```python
from build123d import *

# Parameters (mm, degrees)
SKETCH5_W           = 6.1595
SKETCH5_H           = 101.6
SKETCH5_W_2         = 101.6
SKETCH5_H_2         = 6.1595
BOSS_EXTRUDE1_DEPTH = 19.05
SKETCH6_W           = 333.025633445
SKETCH6_H           = 150.821732437
CUT_EXTRUDE1_DEPTH  = 205.486
SKETCH7_W           = 172.839732196
SKETCH7_H           = 155.996881263
CUT_EXTRUDE2_DEPTH  = 205.486
SKETCH8_W           = 181.528793167
SKETCH8_H           = 183.344081098
CUT_EXTRUDE3_DEPTH  = 147.066


with BuildPart() as part:
    # Sketch2 → Loft1 section 0
    with BuildSketch(Plane(origin=(0, 127, 0), x_dir=(1, 0, 0), z_dir=(0, 1, 0))):
        with BuildLine():
            Line((-50.8, -50.8), (278.13, -50.8))
            Line((278.13, -50.8), (278.13, 276.352))
            Line((278.13, 276.352), (-50.8, 276.352))
            Line((-50.8, 276.352), (-50.8, -50.8))
        make_face()
    # Sketch1 → Loft1 section 1
    with BuildSketch(Plane(origin=(0, 0, 0), x_dir=(1, 0, 0), z_dir=(0, 1, 0))):
        with BuildLine():
            Line((0, 0), (227.33, 0))
            Line((227.33, 0), (227.33, 225.552))
            Line((227.33, 225.552), (0, 225.552))
            Line((0, 225.552), (0, 0))
        make_face()
    loft()

    # Sketch4 → Cut-Loft3 section 0
    with BuildSketch(Plane.XZ):
        with BuildLine():
            Line((208.28, -19.05), (19.05, -19.05))
            Line((19.05, -19.05), (19.05, -206.502))
            Line((19.05, -206.502), (208.28, -206.502))
            Line((208.28, -206.502), (208.28, -19.05))
        make_face()
    # Sketch3 → Cut-Loft3 section 1
    with BuildSketch(Plane(origin=(0, 127, 0), x_dir=(1, 0, 0), z_dir=(0, 1, 0))):
        with BuildLine():
            Line((-31.75, 257.302), (-31.75, -31.75))
            Line((-31.75, -31.75), (259.08, -31.75))
            Line((259.08, -31.75), (259.08, 257.302))
            Line((259.08, 257.302), (-31.75, 257.302))
        make_face()
    loft(mode=Mode.SUBTRACT)

    # Sketch5 → Boss-Extrude1 (add)
    with BuildSketch(Plane.XZ):
        with Locations((3.07975, -112.776)):
            Rectangle(SKETCH5_W, SKETCH5_H)
        with Locations((15.97025, -112.776)):
            Rectangle(SKETCH5_W, SKETCH5_H)
        with Locations((113.665, -3.07975)):
            Rectangle(SKETCH5_W_2, SKETCH5_H_2)
        with Locations((113.665, -15.97025)):
            Rectangle(SKETCH5_W_2, SKETCH5_H_2)
        with Locations((223.36125, -113.665)):
            Rectangle(SKETCH5_W, SKETCH5_H)
        with Locations((210.47075, -113.665)):
            Rectangle(SKETCH5_W, SKETCH5_H)
        with Locations((112.776, -223.36125)):
            Rectangle(SKETCH5_W_2, SKETCH5_H_2)
        with Locations((112.776, -210.47075)):
            Rectangle(SKETCH5_W_2, SKETCH5_H_2)
    extrude(amount=BOSS_EXTRUDE1_DEPTH)

    # Sketch6 → Cut-Extrude1 (cut)
    with BuildSketch(Plane.XY.offset(-113.2205)):
        with Locations((111.617183278, 51.589133782)):
            Rectangle(SKETCH6_W, SKETCH6_H)
    extrude(amount=-CUT_EXTRUDE1_DEPTH, mode=Mode.SUBTRACT)

    # Sketch7 → Cut-Extrude2 (cut)
    with BuildSketch(Plane.ZY.offset(-113.2205)):
        with Locations((-29.906934154, 52.245596061)):
            Rectangle(SKETCH7_W, SKETCH7_H)
    extrude(amount=-CUT_EXTRUDE2_DEPTH, mode=Mode.SUBTRACT)

    # Sketch8 → Cut-Extrude3 (cut)
    with BuildSketch(Plane(origin=(0, 6.35, 0), x_dir=(-1, 0, 0), z_dir=(0, -1, 0))):
        with Locations((-25.634722782, 25.303882613)):
            Rectangle(SKETCH8_W, SKETCH8_H)
    extrude(amount=-CUT_EXTRUDE3_DEPTH, mode=Mode.SUBTRACT)


solid = part.part
```
CAD build for the part. Positions are in the model's coordinates, mm. A direction names the side the tool comes from. Coordinates: 2 decimals unless noted, no trailing zeros. Return JSON: item names as keys, results as strings. Group by question number.
Q1. Cut at A-A, the plane y = -3.25. State how many separate pieces and enclosed holes the cut face has, then the cut area to 3 significant figures.
Q2. Drill centre lines: line 1 (Z direction, x = 100.5, y = -3.25); line 2 (X direction, y = -3.25, z = -69.5); line 3 (Y direction, x = 36, z = -10). Where is each one in solid material? Low to high.
Q3. Flat gauge pins, fed straight in: pin 1 (7 mm diameter, centred on y = -6.5, z = -2.5, fed in from -X) (3 decimals); pin 2 (5 mm diameter, centred on x = 3.5, y = -7.5, fed in from +Z); pin 3 (6 mm diameter, centred on x = 66, y = -4.5, fed in from -Z). Where does each tip first touch, or does it go through?
Q4. Pull direction Z, two halves, no side cores. Call faces 1 (the face through (88, -9, -6.16)), 2 (the face through (12.89, -9, -88)), 3 (the face through (3, -9, -61.976)), 4 (the face through (88, -9, -12.89)): released by +Z, released by -Z, zero draft, split by the parting line, or undercut.
Q5. Which spindle directions (+Z, -Z, +X, -X, +Y, -Y) get a long thin tool onto all of the face, cutting with end or side? Do faces 5 (the face through (6.16, -9, -88)), 6 (the face through (113.22, -6, -6)), 7 (the face through (16, -9, -61.976)), 8 (the face through (3, -19.05, -87)), 9 (the face through (62.865, -9, -16)). Say none if no direction does.
Returned:
{
 "1": {"separate pieces": "4", "enclosed holes": "0", "area": "1,250 mm2"},
 "2": {"line 1": "z = -19.05 to -12.89, -6.16 to 0", "line 2": "x = 0 to 6.16, 12.89 to 19.05", "line 3": "y = 0 to 6.35"},
 "3": {"pin 1": "stops at x = 62.865", "pin 2": "stops at z = -61.98", "pin 3": "stops at z = -19.05"},
 "4": {"face 1": "undercut", "face 2": "zero draft", "face 3": "released by +Z", "face 4": "undercut"},
 "5": {"face 5": "+Z, -Z, -Y", "face 6": "+Z, -Z, +X, +Y, -Y", "face 7": "+Z, +X, -X, -Y", "face 8": "+Z, -Z, +X, -X, -Y", "face 9": "+Z, -Z, -X, -Y"}
}
